```python
from build123d import *

# Parameters (mm, degrees)
SKETCH1_W           = 51
SKETCH1_H           = 22.352
SKETCH1_R           = 1.6
BOSS_EXTRUDE1_DEPTH = 2
SKETCH2_W           = 19
SKETCH2_H           = 7
BOSS_EXTRUDE2_DEPTH = 10.5
SKETCH3_W           = 43.18
SKETCH3_H           = 7.62
BOSS_EXTRUDE3_DEPTH = 4.5


with BuildPart() as part:
    # Sketch1 → Boss-Extrude1 (new body)
    with BuildSketch(Plane(origin=(0, 0, 0), x_dir=(1, 0, 0), z_dir=(0, 1, 0))):
        Rectangle(SKETCH1_W, SKETCH1_H)
        with Locations(Location((22.252, 8.005562403, 0), (0, 0, 270))):
            Circle(SKETCH1_R, mode=Mode.SUBTRACT)
    extrude(amount=BOSS_EXTRUDE1_DEPTH)

    # Sketch2 → Boss-Extrude2 (add)
    with BuildSketch(Plane(origin=(0, 2, 0), x_dir=(1, 0, 0), z_dir=(0, 1, 0))):
        with Locations((16, -7.676)):
            Rectangle(SKETCH2_W, SKETCH2_H)
    extrude(amount=BOSS_EXTRUDE2_DEPTH)

    # Sketch3 → Boss-Extrude3 (add)
    with BuildSketch(Plane.XZ):
        with Locations((-3.91, -7.366)):
            Rectangle(SKETCH3_W, SKETCH3_H)
    extrude(amount=BOSS_EXTRUDE3_DEPTH)


solid = part.part
```
Work out the finished part from the listing and answer in its coordinate system (mm). A direction names the side the tool comes from. Coordinates: 2 decimals unless noted, no trailing zeros. Write each loop counter-clockwise with the first axis right and the second up, starting at its lowest first coordinate (ties: lowest second). Pieces come first, ordered by that corner, then holes.
Q1. A cutting plane is placed at A-A, the plane z = -7.5. Give the vertices of the cut face in (x, y), then the cut area to 3 significant figures.
Q2. Determine the mould class of faces 4 (the face through (16, 12.5, 8)), 5 (the face through (11, 5, 11.176)), 6 (the face through (0, -1, -11.176)), 7 (the face through (22.322, 0.986, -9.604)) for opening direction Z: released by +Z, released by -Z, zero draft, split by the parting line, or undercut.
Q3. Each of these flat-tipped pins is pushed along its axis until it touches: pin 1 Ø5 at (x, y) = (4.5, -1.5) entering from +Z; pin 2 Ø1 at (y, z) = (4.5, 6) entering from -X; pin 3 Ø3.5 at (y, z) = (-3, -6) entering from +X; pin 4 Ø4 at (x, z) = (22.25, -8.01) entering from -Y. Where does it stop, or does it pass through?
Q4. A cutting plane is placed at D-D, the plane z = 6.25. Give the vertices of the cut face in (x, y), then the cut area to 4 significant figures.
Q5. Which of the six approach directions +Z, -Z, +X, -X, +Y, -Y give full straight-line access (tool end or side, diameter ignored) to faces 1 (the face through (16, 7, 4.176)), 2 (the face through (6.5, 7, 8)), 3 (the face through (17.68, -2, -7))?
Q6. A cutting plane is placed at B-B, the plane x = 18.5. Give the vertices of the cut face in (y, z), then the cut area to 3 significant figures.
Q7. Find the intervals of material crossed by line 1 (Y direction, x = 0, z = -9.75); line 2 (Y direction, x = -13, z = 3.25); line 3 (Z direction, x = 10, y = 9.75), in increasing order.
Q8. A cutting plane is placed at C-C, the plane y = 10.75. Give the vertices of the cut face in (x, z), then the cut area to 3 significant figures.
Findings below:
1. outline: (-25.5, -4.5) - (17.68, -4.5) - (17.68, 0) - (20.73, 0) - (20.73, 2) - (-25.5, 2) - close; (23.77, 0) - (25.5, 0) - (25.5, 2) - (23.77, 2) - close
1. area: 290 mm2
2. face 4: zero draft
2. face 5: released by +Z
2. face 6: released by -Z
2. face 7: undercut
3. pin 1: stops at z = 11.18
3. pin 2: stops at x = 6.5
3. pin 3: stops at x = 17.68
3. pin 4: stops at y = 0
4. outline: (-25.5, 0) - (25.5, 0) - (25.5, 12.5) - (6.5, 12.5) - (6.5, 2) - (-25.5, 2) - close
4. area: 301.5 mm2
5. face 1: -Z, +X, -X, +Y
5. face 2: +Z, -Z, -X, +Y
5. face 3: +Z, -Z, +X, -Y
6. outline: (0, -11.18) - (2, -11.18) - (2, 4.18) - (12.5, 4.18) - (12.5, 11.18) - (0, 11.18) - close
6. area: 118 mm2
7. line 1: y = -4.5 to 2
7. line 2: y = 0 to 2
7. line 3: z = 4.18 to 11.18
8. outline: (6.5, 4.18) - (25.5, 4.18) - (25.5, 11.18) - (6.5, 11.18) - close
8. area: 133 mm2
